```python
from build123d import *

# Parameters (mm, degrees)
SKETCH1_W           = 32
SKETCH1_H           = 144
BOSS_EXTRUDE1_DEPTH = 15
SKETCH2_R           = 18
BOSS_EXTRUDE2_DEPTH = 14
SKETCH3_R           = 16
BOSS_EXTRUDE3_DEPTH = 14
SKETCH4_R           = 8.25
CUT_EXTRUDE1_DEPTH  = 216.278888886
SKETCH5_R           = 7
BOSS_EXTRUDE4_DEPTH = 20
SKETCH6_R           = 10
CUT_EXTRUDE2_DEPTH  = 216.684955433


with BuildPart() as part:
    # Sketch1 → Boss-Extrude1 (new, symmetric)
    with BuildSketch(Plane.XY):
        with Locations((0, 136)):
            Rectangle(SKETCH1_W, SKETCH1_H)
    extrude(amount=BOSS_EXTRUDE1_DEPTH, both=True)

    # Sketch2 → Boss-Extrude2 (add, symmetric)
    with BuildSketch(Plane.XY):
        with Locations((0, 76)):
            Circle(SKETCH2_R)
    extrude(amount=BOSS_EXTRUDE2_DEPTH, both=True)

    # Sketch3 → Boss-Extrude3 (add, symmetric)
    with BuildSketch(Plane.XY):
        with Locations((0, 198)):
            Circle(SKETCH3_R)
    extrude(amount=BOSS_EXTRUDE3_DEPTH, both=True)

    # Sketch4 → Cut-Extrude1 (cut, through all)
    with BuildSketch(Plane.XY):
        with Locations((0, 76)):
            Circle(SKETCH4_R)
    extrude(amount=-CUT_EXTRUDE1_DEPTH, mode=Mode.SUBTRACT)

    # Sketch5 → Boss-Extrude4 (add, symmetric)
    with BuildSketch(Plane.XY):
        with Locations(Location((0, 198, 0), (0, 0, 180))):
            Circle(SKETCH5_R)
    extrude(amount=BOSS_EXTRUDE4_DEPTH, both=True)

    # Sketch6 → Cut-Extrude2 (cut, through all)
    with BuildSketch(Plane.XY):
        with Locations((0, 118)):
            Circle(SKETCH6_R)
        with Locations((0, 155)):
            Circle(SKETCH6_R)
    extrude(amount=-CUT_EXTRUDE2_DEPTH, mode=Mode.SUBTRACT)


solid = part.part
```
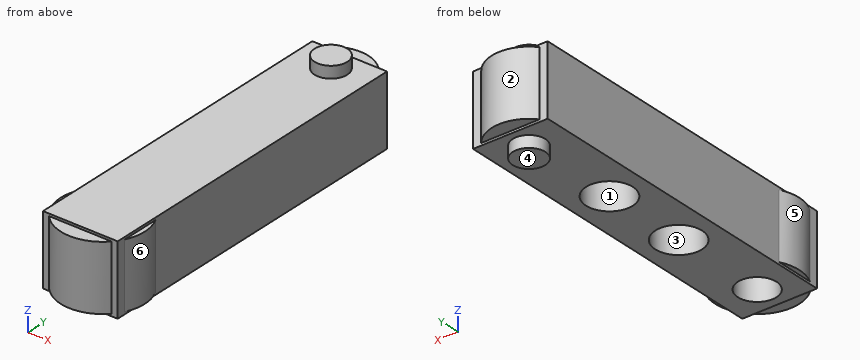
Input: part model. Units: mm. Frame: model coordinates. Face numbers are marked on the shaded views. A direction names the side the tool comes from. Give positions to 0.01 mm unless a question says otherwise; leave off trailing zeros. Write each loop counter-clockwise with the first axis right and the second up, starting at its lowest first coordinate (ties: lowest second). Pieces come first, ordered by that corner, then holes. Notation, with made-up numbers: (43, -0.75) - (83, -0.75) arc R22 ccw to (83, 24.25) - close; hole circle Ø4 at (7.5, -38). An arc over 180 degrees is marked (long way). Write item = value, one per line. Start each with the question number.
1. Ray query, L1, parallel to Y at x = -0.5, z = -3.5; L2, parallel to Y at x = -1.5, z = -11.5; L3, parallel to X at y = 95, z = -4. Return the intervals inside material, ascending.
2. Access query for the marked faces 1 and 2. Directions: +Z, -Z, +X, -X, +Y, -Y. A direction counts if a zero-diameter tool reaches every point of the face in a straight line with its end or side. Return the directions, or none.
3. Mould query, pull axis X, two halves, no side actions, for the marked faces 3, 4, 5 and 6. Classes: released by +X, released by -X, zero draft, split by the parting line, or undercut.
4. Section query D-D, the plane y = 198. Output: boundary loops of the cut face in (x, z).
5. First-contact query: pin 1 Ø12 at (x, y) = (0, 118) entering from +Z; pin 2 Ø1 at (x, y) = (17.5, 78.5) entering from -Z; pin 3 Ø15 at (y, z) = (117.5, -3) entering from +X. Flat tips, straight axial feed; report the tip coordinate or a pass-through.
6. Section query B-B, the plane y = 118. Output: boundary loops of the cut face in (x, z).
7. Section query A-A, the plane z = -1.5. Output: boundary loops of the cut face in (x, y), then the cut area to 3 significant figures.
Check sheet entries:
q1.L1 = 58.01 to 67.77, 84.23 to 108.01, 127.99 to 145.01, 164.99 to 213.99
q1.L2 = 58.06 to 67.89, 84.11 to 108.11, 127.89 to 145.11, 164.89 to 213.93
q1.L3 = -16 to 16
q2.face_1 = -Z
q2.face_2 = +Z, -Z, +Y
q3.face_3 = undercut
q3.face_4 = zero draft
q3.face_5 = released by -X
q3.face_6 = released by +X
q4.outline = (-16, -15) - (-7, -15) - (-7, -20) - (7, -20) - (7, -15) - (16, -15) - (16, 15) - (7, 15) - (7, 20) - (-7, 20) - (-7, 15) - (-16, 15) - close
q5.pin_1 = 15
q5.pin_2 = -14
q5.pin_3 = 16
q6.outline = (-16, -15) - (-10, -15) - (-10, 0) - (10, 0) - (10, -15) - (16, -15) - (16, 15) - (-16, 15) - close
q7.outline = (-16, 64) - (-13.42, 64) arc R18 ccw to (13.42, 64) - (16, 64) - (16, 67.75) arc R18 ccw to (16, 84.25) - (16, 208) - (12.49, 208) arc R16 ccw to (-12.49, 208) - (-16, 208) - (-16, 84.25) arc R18 ccw to (-16, 67.75) - close; hole circle Ø20 at (0, 118); hole circle Ø20 at (0, 155); hole circle Ø16.5 at (0, 76)
q7.area = 4,030 mm2
